```python
from build123d import *

# Parameters (mm, degrees)
BOSS_EXTRUDE1_DEPTH = 1.524


with BuildPart() as part:
    # Sketch1 → Boss-Extrude1 (new body)
    with BuildSketch(Plane.XY):
        with BuildLine():
            Line((-0.762799401, 4.151739841), (0.763181799, 4.152733255))
            Line((0.763181799, 4.152733255), (0.763181799, 1.101764269))
            ThreePointArc((0.763181799, 1.101764269), (4.319640518, 0.186449021), (6.371385502, -2.859292784))
            ThreePointArc((6.371385502, -2.859292784), (6.672574584, -10.435641577), (4.151071361, -17.586431561))
            ThreePointArc((4.151071361, -17.586431561), (3.785308505, -19.389837846), (4.258503872, -21.168079349))
            ThreePointArc((4.258503872, -21.168079349), (4.695327747, -19.753303526), (5.694864831, -18.660906461))
            ThreePointArc((5.694864831, -18.660906461), (9.578008584, -11.987204881), (10.914606675, -4.382561317))
            ThreePointArc((10.914606675, -4.382561317), (11.963687789, -1.143514723), (11.54368289, 2.235181758))
            ThreePointArc((11.54368289, 2.235181758), (11.063913724, 1.182736218), (10.240953414, 0.369990013))
            ThreePointArc((10.240953414, 0.369990013), (9.378846201, 3.251271559), (8.129251062, 5.986874633))
            ThreePointArc((8.129251062, 5.986874633), (7.646964471, 7.353540521), (7.350228625, 8.772104529))
            ThreePointArc((7.350228625, 8.772104529), (7.140948693, 8.388008696), (6.822386333, 8.088265938))
            ThreePointArc((6.822386333, 8.088265938), (6.395648788, 8.676833831), (5.949561914, 9.25087529))
            ThreePointArc((5.949561914, 9.25087529), (2.381070398, 14.85503863), (0.00144629, 21.058115893))
            ThreePointArc((0.00144629, 21.058115893), (-2.237613904, 14.848855853), (-5.874078491, 9.34027835))
            ThreePointArc((-5.874078491, 9.34027835), (-6.359611605, 8.722749648), (-6.822768731, 8.088265938))
            ThreePointArc((-6.822768731, 8.088265938), (-7.141331091, 8.388008696), (-7.350611023, 8.772104529))
            ThreePointArc((-7.350611023, 8.772104529), (-7.647346869, 7.353540521), (-8.12963346, 5.986874633))
            ThreePointArc((-8.12963346, 5.986874633), (-9.386584799, 3.258077765), (-10.259685397, 0.383368325))
            ThreePointArc((-10.259685397, 0.383368325), (-11.070398481, 1.192598639), (-11.54368289, 2.235724362))
            ThreePointArc((-11.54368289, 2.235724362), (-11.954593886, -1.23311659), (-10.820946706, -4.537136787))
            ThreePointArc((-10.820946706, -4.537136787), (-9.502375995, -12.050586646), (-5.695247229, -18.660906461))
            ThreePointArc((-5.695247229, -18.660906461), (-4.695710145, -19.753303526), (-4.25888627, -21.168079349))
            ThreePointArc((-4.25888627, -21.168079349), (-3.785690903, -19.389837846), (-4.151453759, -17.586431561))
            ThreePointArc((-4.151453759, -17.586431561), (-6.675465031, -10.434527086), (-6.375410647, -2.856246417))
            ThreePointArc((-6.375410647, -2.856246417), (-4.320748698, 0.188135712), (-0.762909272, 1.100098915))
            Line((-0.762909272, 1.100098915), (-0.762799401, 4.151739841))
        make_face()
    extrude(amount=BOSS_EXTRUDE1_DEPTH)


solid = part.part
```
Design review of the part built by this model. Coordinates are the model's own, in mm. A direction names the side the tool comes from. Round coordinates to 2 decimals unless told otherwise and drop trailing zeros. Write each loop counter-clockwise with the first axis right and the second up, starting at its lowest first coordinate (ties: lowest second). Pieces come first, ordered by that corner, then holes.
Item 1: For probe 1 along X at (y, z) = (-13.5, 0.6); probe 2 along X at (y, z) = (-12, 0.8); probe 3 along Y at (x, z) = (-3.25, 0.7), list the stretches that pass through material, from the lowest coordinate up.
Item 2: The part is to be moulded in two halves that separate along X. For faces 1 (the cylindrical face through (-2.196, 14.932, 0.751)), 2 (the cylindrical face through (-9.37, 3.3, 0.75)), 3 (the cylindrical face through (11.96, -1.19, 0.75)), 4 (the cylindrical face through (-6.66, -10.54, 0.75)), say which applies: +X half, -X half, draft (parallel to the pull), parting line (faces both ways), or undercut.
Item 3: For faces 5 (the cylindrical face through (-6.353, 8.732, 0.751)), 6 (the flat face through (0, 5, 0)), 7 (the cylindrical face through (4.3, 0.2, 0.8)), 8 (the flat face through (0.763, 3, 1)), 9 (the flat face through (0, 5, 1.524)), list the 3-axis set-ups (+Z, -Z, +X, -X, +Y, -Y) from which the entire face can be reached by the end or side of a thin tool; tool diameter is ignored.
Item 4: We need section A-A on y = -6.5. Write out the cut boundary in (x, z).
Item 5: We need section C-C on x = -3. Write out the cut boundary in (y, z), and give its area (3 significant figures).
Item 6: We need section B-B on z = 1. Write out the cut boundary in (x, y), and give its area (3 significant figures).
Item 7: Clearance check with a flat-ended pin moving along its axis: pin 1 Ø5 at (x, y) = (-0.5, 9) entering from -Z. State where the tip first meets the part, or that it passes through.
Item 8: We need section D-D on y = -12. Write out the cut boundary in (x, z), and give its area (3 significant figures).
Returned:
1. probe 1: x = -8.92 to -5.96, 5.96 to 8.96
1. probe 2: x = -9.52 to -6.38, 6.37 to 9.57
1. probe 3: y = 0.77 to 13.01
2. face 1: -X half
2. face 2: undercut
2. face 3: +X half
2. face 4: undercut
3. face 5: +Z, -Z, +Y
3. face 6: -Z, +X, -X, +Y, -Y
3. face 7: +Z, -Z
3. face 8: +Z, -Z, -Y
3. face 9: +Z, +X, -X, +Y, -Y
4. outline: (-10.73, 0) - (-6.88, 0) - (-6.88, 1.52) - (-10.73, 1.52) - close; (6.88, 0) - (10.82, 0) - (10.82, 1.52) - (6.88, 1.52) - close
5. outline: (0.86, 0) - (13.43, 0) - (13.43, 1.52) - (0.86, 1.52) - close
5. area: 19.2 mm2
6. outline: (-11.54, 2.24) arc R7.86 ccw to (-10.82, -4.54) arc R21.98 ccw to (-5.7, -18.66) arc R3.38 cw to (-4.26, -21.17) arc R4.03 ccw to (-4.15, -17.59) arc R20.14 cw to (-6.38, -2.86) arc R5.17 cw to (-0.76, 1.1) - (-0.76, 4.15) - (0.76, 4.15) - (0.76, 1.1) arc R5.17 cw to (6.37, -2.86) arc R20.14 cw to (4.15, -17.59) arc R4.03 ccw to (4.26, -21.17) arc R3.38 cw to (5.69, -18.66) arc R21.99 ccw to (10.91, -4.38) arc R7.86 ccw to (11.54, 2.24) arc R3.2 cw to (10.24, 0.37) arc R21.85 ccw to (8.13, 5.99) arc R10.9 cw to (7.35, 8.77) arc R1.39 cw to (6.82, 8.09) arc R21.84 ccw to (5.95, 9.25) arc R33.16 cw to (0, 21.06) arc R27.87 cw to (-5.87, 9.34) arc R21.98 ccw to (-6.82, 8.09) arc R1.39 cw to (-7.35, 8.77) arc R10.9 cw to (-8.13, 5.99) arc R21.98 ccw to (-10.26, 0.38) arc R3.2 cw to start
6. area: 355 mm2
7. pin 1: stops at z = 0
8. outline: (-9.52, 0) - (-6.38, 0) - (-6.38, 1.52) - (-9.52, 1.52) - close; (6.37, 0) - (9.57, 0) - (9.57, 1.52) - (6.37, 1.52) - close
8. area: 9.67 mm2
